```python
from build123d import *

# Parameters (mm, degrees)
F1_DEPTH = 25.4
F3_DEPTH = 12.7
F5_DEPTH = 12.7


with BuildPart() as f1:
    # F0 (on Right) → F1 (new body, symmetric)
    with BuildSketch(Plane.YZ):
        Polygon((-30.7642482221, 59.8066113889), (-43.1617796421, 62.7912059426), (-38.7996844947, -26.0577760637), (36.5038476884, -26.0577760637), (51.6563877463, -3.328967141), (-18.8258830458, 0), align=None)
    extrude(amount=F1_DEPTH, both=True)

    # F2 (on face) → F3 (join)
    with BuildSketch(Plane.YZ.offset(25.4)):
        with BuildLine():
            Line((-38.7996844947, -26.0577760637), (-39.9597344248, -2.4293929413))
            ThreePointArc((-39.9597344248, -2.4293929413), (-43.9297710113, -33.6056919757), (-13.4215462618, -26.0577760637))
            Line((-13.4215462618, -26.0577760637), (-38.7996844947, -26.0577760637))
        make_face()
        with BuildLine():
            ThreePointArc((23.0047428651, -1.9757135742), (14.2789928232, -12.4410495521), (14.7757120925, -26.0577760637))
            Line((14.7757120925, -26.0577760637), (36.5038476884, -26.0577760637))
            Line((36.5038476884, -26.0577760637), (48.3362770566, -8.3091329206))
            ThreePointArc((48.3362770566, -8.3091329206), (46.0012077103, -5.3595465788), (43.1320322619, -2.9263510081))
            Line((43.1320322619, -2.9263510081), (23.0047428651, -1.9757135742))
        make_face()
        with BuildLine():
            Line((36.5038476884, -26.0577760637), (14.7757120925, -26.0577760637))
            ThreePointArc((14.7757120925, -26.0577760637), (36.1107346383, -37.2669929283), (51.3556094348, -18.6008866876))
            ThreePointArc((51.3556094348, -18.6008866876), (50.585198027, -13.2381317144), (48.3362770566, -8.3091329206))
            Line((48.3362770566, -8.3091329206), (36.5038476884, -26.0577760637))
        make_face()
        with BuildLine():
            ThreePointArc((43.1320322619, -2.9263510081), (33.2043632144, 0.427900495), (23.0047428651, -1.9757135742))
            Line((23.0047428651, -1.9757135742), (43.1320322619, -2.9263510081))
        make_face()
        with BuildLine():
            ThreePointArc((-13.4215462618, -26.0577760637), (-12.5168247449, -22.7721507415), (-12.2119991601, -19.3779002875))
            ThreePointArc((-12.2119991601, -19.3779002875), (-21.3319779313, -3.1206810174), (-39.9597344248, -2.4293929413))
            Line((-39.9597344248, -2.4293929413), (-38.7996844947, -26.0577760637))
            Line((-38.7996844947, -26.0577760637), (-13.4215462618, -26.0577760637))
        make_face()
    extrude(amount=F3_DEPTH)

    # F4 (on face) → F5 (join)
    with BuildSketch(Plane(origin=(-25.4, 0, 0), x_dir=(0, -1, 0), z_dir=(-1, 0, 0))):
        with BuildLine():
            ThreePointArc((-49.9511753023, -5.886785676), (-44.364371435, -32.8563377087), (-17.6745105539, -26.0577760637))
            Line((-17.6745105539, -26.0577760637), (-36.5038476884, -26.0577760637))
            Line((-36.5038476884, -26.0577760637), (-49.9511753023, -5.886785676))
        make_face()
        with BuildLine():
            ThreePointArc((-17.6745105539, -26.0577760637), (-15.8427926815, -21.5381365786), (-15.2185845072, -16.7015369886))
            ThreePointArc((-15.2185845072, -16.7015369886), (-17.0599821691, -8.5304596075), (-22.2281913909, -1.9390360621))
            Line((-22.2281913909, -1.9390360621), (-47.6467773495, -3.1395881509))
            ThreePointArc((-47.6467773495, -3.1395881509), (-48.8637569956, -4.4588477401), (-49.9511753023, -5.886785676))
            Line((-49.9511753023, -5.886785676), (-36.5038476884, -26.0577760637))
            Line((-36.5038476884, -26.0577760637), (-17.6745105539, -26.0577760637))
        make_face()
        with BuildLine():
            Line((-47.6467773495, -3.1395881509), (-22.2281913909, -1.9390360621))
            ThreePointArc((-22.2281913909, -1.9390360621), (-35.1673382867, 2.3272501941), (-47.6467773495, -3.1395881509))
        make_face()
        with BuildLine():
            ThreePointArc((39.9746132614, -2.1263345619), (19.3411728577, -5.6965682778), (14.4517302333, -26.0577760637))
            Line((14.4517302333, -26.0577760637), (38.7996844947, -26.0577760637))
            Line((38.7996844947, -26.0577760637), (39.9746132614, -2.1263345619))
        make_face()
        with BuildLine():
            Line((38.7996844947, -26.0577760637), (14.4517302333, -26.0577760637))
            ThreePointArc((14.4517302333, -26.0577760637), (35.6526480592, -38.358509601), (51.4213347316, -19.5932362791))
            ThreePointArc((51.4213347316, -19.5932362791), (48.3047109587, -9.151492076), (39.9746132614, -2.1263345619))
            Line((39.9746132614, -2.1263345619), (38.7996844947, -26.0577760637))
        make_face()
    extrude(amount=F5_DEPTH)


solid = f1.part
```
The model under review builds one solid part; all positions refer to its coordinate system, in mm. A direction names the side the tool comes from. Round coordinates to 2 decimals unless told otherwise and drop trailing zeros. Write each loop counter-clockwise with the first axis right and the second up, starting at its lowest first coordinate (ties: lowest second). Pieces come first, ordered by that corner, then holes.
(1) We need section A-A on y = -24.5. Give the boundary of the cut face in (x, z), and give its area (3 significant figures).
(2) Machinability: for faces 1 (the flat face through (25.4, 33, -1)), 2 (the flat face through (-25.4, 50, -4)), 3 (the flat face through (25.4, 37, -26)), 4 (the flat face through (25.4, -36, -28)), which of the approach directions +Z, -Z, +X, -X, +Y, -Y give a long, thin tool a straight path to every point of the face, cutting with its end or side? Answer none if there is none.
(3) Wall thickness on L1, parallel to X at y = -42.5, z = -17; L2, parallel to X at y = 27, z = 0.5; L3, parallel to X at y = -30, z = 20.5: over which ranges is each line inside the solid? List them lowest first.
(4) We need section B-B on z = -21. Give the boundary of the cut face in (x, y).
(5) We need section C-C on x = -24. Give the boundary of the cut face in (y, z), and give its area (3 significant figures).
(6) We need section D-D on y = 19. Give the boundary of the cut face in (x, z).
(7) Insertion check: pin 1 (8 mm diameter, centred on x = 28, z = -3.5, fed in from -Y); pin 2 (6 mm diameter, centred on x = 25.5, z = -17.5, fed in from +Y); pin 3 (1.5 mm diameter, centred on x = 4, z = -21.5, fed in from +Y). Each pin has a flat end and moves straight along its axis. Give the tip position at first contact, or say it passes through.
(8) Mouldability with a two-part tool opening along X and no side actions: class faces 5 (the flat face through (0, -2, -26.058)), 6 (the flat face through (0.36, -36.88, 61.28)), 7 (the flat face through (25.4, -22, 5)) as +X half, -X half, draft (parallel to the pull), parting line (faces both ways), or undercut.
Findings below:
1. outline: (-38.1, -36.94) - (-25.4, -36.94) - (-25.4, -26.06) - (25.4, -26.06) - (25.4, -37.19) - (38.1, -37.19) - (38.1, -1.57) - (25.4, -1.57) - (25.4, 28.43) - (-25.4, 28.43) - (-25.4, -2.25) - (-38.1, -2.25) - close
1. area: 3,660 mm2
2. face 1: +Z, +Y
2. face 2: +Z, -X, +Y
2. face 3: -Z, +Y
2. face 4: -Z, -Y
3. L1: x = -38.1 to -25.4, 25.4 to 38.1
3. L2: x = -38.1 to -25.4
3. L3: x = -25.4 to 25.4
4. outline: (-38.1, -51.37) - (-25.4, -51.37) - (-25.4, -39.05) - (25.4, -39.05) - (25.4, -50.24) - (38.1, -50.24) - (38.1, -12.28) - (25.4, -12.28) - (25.4, 13.41) - (38.1, 13.41) - (38.1, 51.2) - (25.4, 51.2) - (25.4, 39.88) - (-25.4, 39.88) - (-25.4, 52.83) - (-38.1, 52.83) - (-38.1, 15.71) - (-25.4, 15.71) - (-25.4, -13.37) - (-38.1, -13.37) - close
5. outline: (-43.16, 62.79) - (-38.8, -26.06) - (36.5, -26.06) - (51.66, -3.33) - (-18.83, 0) - (-30.76, 59.81) - close
5. area: 3,100 mm2
6. outline: (-38.1, -28.09) - (-25.4, -28.09) - (-25.4, -26.06) - (25.4, -26.06) - (25.4, -32.23) - (38.1, -32.23) - (38.1, -4.97) - (25.4, -4.97) - (25.4, -1.79) - (-25.4, -1.79) - (-25.4, -5.31) - (-38.1, -5.31) - close
7. pin 1: stops at y = -46.16
7. pin 2: stops at y = 51.36
7. pin 3: stops at y = 40.04
8. face 5: undercut
8. face 6: draft
8. face 7: +X half
